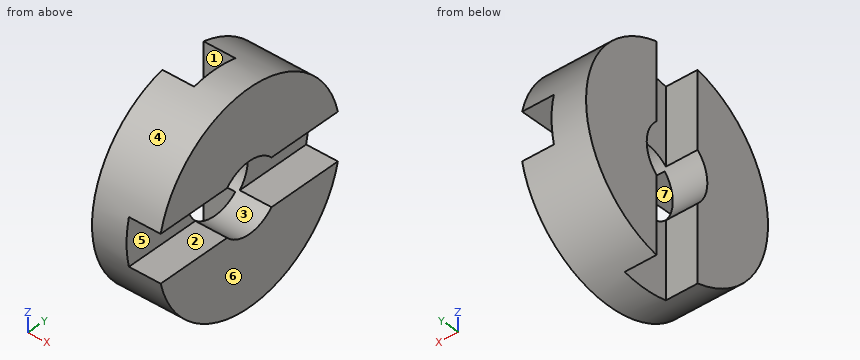
```python
from build123d import *

# Parameters (mm, degrees)
SKETCH1_W               = 4.8
SKETCH1_H               = 5
SKETCH2_W               = 2.3
SKETCH2_H               = 3.4
CUT_EXTRUDE1_DEPTH      = 7.5
CUT_EXTRUDE1_DEPTH_BACK = 7.5
SKETCH3_W               = 2.3
SKETCH3_H               = 3.4
CUT_EXTRUDE2_DEPTH      = 7.5
CUT_EXTRUDE2_DEPTH_BACK = 7.5


with BuildPart() as part:
    # Sketch1 → Revolve1 (revolve)
    with BuildSketch(Plane.XY):
        with Locations((2.4, 5)):
            Rectangle(SKETCH1_W, SKETCH1_H)
    revolve(axis=Axis((4.8, 0, 0), (-1, 0, 0)))

    # Sketch2 → Cut-Extrude1 (cut, two sides)
    with BuildSketch(Plane.XY) as cut_extrude1_sk:
        with Locations((1.15, 0)):
            Rectangle(SKETCH2_W, SKETCH2_H)
    extrude(amount=CUT_EXTRUDE1_DEPTH, mode=Mode.SUBTRACT)
    extrude(cut_extrude1_sk.sketch, amount=-CUT_EXTRUDE1_DEPTH_BACK, mode=Mode.SUBTRACT)

    # Sketch3 → Cut-Extrude2 (cut, two sides)
    with BuildSketch(Plane(origin=(0, 0, 0), x_dir=(-1, 0, 0), z_dir=(0, 1, 0))) as cut_extrude2_sk:
        with Locations((-3.65, 0)):
            Rectangle(SKETCH3_W, SKETCH3_H)
    extrude(amount=CUT_EXTRUDE2_DEPTH, mode=Mode.SUBTRACT)
    extrude(cut_extrude2_sk.sketch, amount=-CUT_EXTRUDE2_DEPTH_BACK, mode=Mode.SUBTRACT)


solid = part.part
```
Input: part model. Units: mm. Frame: model coordinates. Face numbers are marked on the shaded views. A direction names the side the tool comes from. Give positions to 0.01 mm unless a question says otherwise; leave off trailing zeros. Write each loop counter-clockwise with the first axis right and the second up, starting at its lowest first coordinate (ties: lowest second). Pieces come first, ordered by that corner, then holes. Notation, with made-up numbers: (6.5, -33) - (58.5, -33) arc R8 ccw to (58.5, -24) - close; hole circle Ø8 at (48, 26.25). An arc over 180 degrees is marked (long way). Write item = value, one per line. Start each with the question number.
1. Mould query, pull axis Z, two halves, no side actions, for the marked faces 4, 5, 6 and 7. Classes: released by +Z, released by -Z, zero draft, split by the parting line, or undercut.
2. Section query C-C, the plane y = -3.75. Output: boundary loops of the cut face in (x, z).
3. Section query A-A, the plane y = 0. Output: boundary loops of the cut face in (x, z), then the cut area to 3 significant figures.
4. First-contact query: pin 1 Ø2.5 at (x, y) = (4, 5.5) entering from +Z; pin 2 Ø0.7 at (x, y) = (3.5, -3.5) entering from +Z; pin 3 Ø1.2 at (x, z) = (0.5, -3.5) entering from +Y. Flat tips, straight axial feed; report the tip coordinate or a pass-through.
5. Section query D-D, the plane z = 5. Output: boundary loops of the cut face in (x, y), then the cut area to 3 significant figures.
6. Section query B-B, the plane z = 0. Output: boundary loops of the cut face in (x, y).
7. Access query for the marked faces 1, 2 and 3. Directions: +Z, -Z, +X, -X, +Y, -Y. A direction counts if a zero-diameter tool reaches every point of the face in a straight line with its end or side. Return the directions, or none.
8. Ray query, L1, parallel to Z at x = 2.8, y = 0; L2, parallel to Z at x = 4.05, y = -3.25; L3, parallel to Y at x = 1.3, z = 0.25. Return the intervals inside material, ascending.
Check sheet entries:
q1.face_4 = split by the parting line
q1.face_5 = undercut
q1.face_6 = zero draft
q1.face_7 = undercut
q2.outline = (0, -6.5) - (4.8, -6.5) - (4.8, -1.7) - (2.5, -1.7) - (2.5, 1.7) - (4.8, 1.7) - (4.8, 6.5) - (0, 6.5) - close
q3.outline = (2.3, -7.5) - (4.8, -7.5) - (4.8, -2.5) - (2.3, -2.5) - close; (2.3, 2.5) - (4.8, 2.5) - (4.8, 7.5) - (2.3, 7.5) - close
q3.area = 25.0 mm2
q4.pin_1 = 6.18
q4.pin_2 = 6.81
q4.pin_3 = 6.92
q5.outline = (0, -5.59) - (4.8, -5.59) - (4.8, 5.59) - (0, 5.59) - (0, 1.7) - (2.3, 1.7) - (2.3, -1.7) - (0, -1.7) - close
q5.area = 45.8 mm2
q6.outline = (0, -7.5) - (2.5, -7.5) - (2.5, -2.5) - (0, -2.5) - close; (0, 2.5) - (2.5, 2.5) - (2.5, 7.5) - (0, 7.5) - close
q7.face_1 = +Z, -Z, -X
q7.face_2 = +X, +Y, -Y
q7.face_3 = +X, -X
q8.L1 = -7.5 to -2.5, 2.5 to 7.5
q8.L2 = -6.76 to -1.7, 1.7 to 6.76
q8.L3 = -7.5 to -2.49, 2.49 to 7.5
